Geometry check sheet. Reference: the model listing, model coordinates, mm. Face numbers are marked on the shaded views. Give positions to 0.01 mm unless a question says otherwise; leave off trailing zeros. Loops run counter-clockwise (first coordinate to the right, second up) from the corner with the lowest first, then second, coordinate; pieces in that order, holes last. Notation, with made-up numbers: (-36.5, -19.75) -> (-32.5, -19.75) arc R25 cw to (-32.5, -1.75) -> close; hole circle Ø1 at (-7, 58.25). An arc over 180 degrees is marked (long way). Answer as a JSON object with one key per item and string values.
from build123d import *

# Parameters (mm, degrees)
F0_W      = 59.395711869
F0_H      = 250.2426505089
F1_DEPTH  = 67.4364492297
F2_R      = 17.4264129212
F3_DEPTH  = 222.8358983994
F4_W      = 62.507584691
F4_H      = 75.5731239915
F5_DEPTH  = 227.648139
F6_W      = 115.2810156345
F6_H      = 19.8185071349
F7_DEPTH  = 53.9569482207
F8_W      = 67.4364492297
F8_H      = 12.6657411456
F8_H_2    = 15.0272101164
F9_DEPTH  = 599.2090702057
F10_R     = 17.5883740648
F11_DEPTH = 151.8874019384
F12_R     = 10.9031193455
F13_DEPTH = 69.4709941745


# Not quite as in the source:
# - a feature names something its author has since deleted; it is built from what else it names


with BuildPart() as f1:
    # F0 (on Front) → F1 (new body)
    with BuildSketch(Plane.XZ):
        Rectangle(F0_W, F0_H)
    extrude(amount=F1_DEPTH)

    # F2 (on face) → F3 (join)
    with BuildSketch(Plane.XY.offset(125.1213252544)):
        with Locations((0, -33.2162864506)):
            Circle(F2_R)
    extrude(amount=-F3_DEPTH)

    # F4 (on face) → F5 (join)
    with BuildSketch(Plane(origin=(-29.6978559345, 0, 0), x_dir=(0, -1, 0), z_dir=(-1, 0, 0))):
        with Locations((36.1826568842, 0)):
            Rectangle(F4_W, F4_H)
    extrude(amount=F5_DEPTH)

    # F6 (on face) → F7 (join)
    with BuildSketch(Plane(origin=(0, -4.9288645387, 0), x_dir=(-1, 0, 0), z_dir=(0, 1, 0))):
        with Locations((168.05139184, 0)):
            Rectangle(F6_W, F6_H)
    extrude(amount=F7_DEPTH)

    # F8 (on face) → F9 (join)
    with BuildSketch(Plane.YZ.offset(29.6978559345)):
        with Locations((-33.7182246149, -118.7884546816)):
            Rectangle(F8_W, F8_H)
        with Locations((-33.7182246149, 117.6077201962)):
            Rectangle(F8_W, F8_H_2)
    extrude(amount=F9_DEPTH)

    # F10 (on face) → F11 (join)
    with BuildSketch(Plane(origin=(-257.3459949344, 0, 0), x_dir=(0, -1, 0), z_dir=(-1, 0, 0))):
        with Locations((40.5630767345, 0)):
            Circle(F10_R)
    extrude(amount=F11_DEPTH)

    # F12 (on face) → F13 (join)
    with BuildSketch(Plane(origin=(0, 0, -9.9092535675), x_dir=(1, 0, 0), z_dir=(0, 0, -1))):
        with Locations((-176.2370765209, -20.2873200178)):
            Circle(F12_R)
    extrude(amount=F13_DEPTH)


solid = f1.part
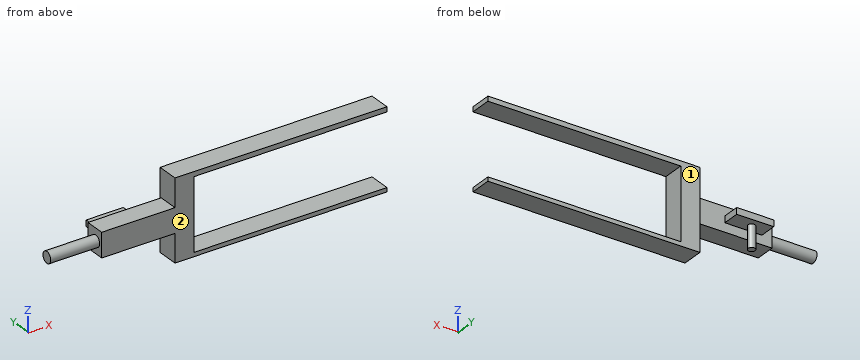
1) Section check B-B on x = -147.5. Record the cut outline in (y, z), plus the area to 3 significant figures.
Geometry check:
{"outline": "(-67.44, -37.79) -> (-4.93, -37.79) -> (-4.93, -9.91) -> (49.03, -9.91) -> (49.03, 9.91) -> (-4.93, 9.91) -> (-4.93, 37.79) -> (-67.44, 37.79) -> close", "area": "5,790 mm2"}
2) Section check C-C on z = 0. Record the cut outline in (x, y), plus the area to 3 significant figures.
Geometry check:
{"outline": "(-409.23, -58.15) -> (-257.35, -58.15) -> (-257.35, -67.44) -> (29.7, -67.44) -> (29.7, 0) -> (-29.7, 0) -> (-29.7, -4.93) -> (-110.41, -4.93) -> (-110.41, 49.03) -> (-225.69, 49.03) -> (-225.69, -4.93) -> (-257.35, -4.93) -> (-257.35, -22.97) -> (-409.23, -22.97) -> close", "area": "29,800 mm2"}
3) Depth check by flat-ended pin: P1, Ø8, axis at x = -149, y = -18.5, coming from the -Z side; P2, Ø4, axis at y = -30, z = 67.5, coming from the -X side; P3, Ø22, axis at y = 22, z = 3, coming from the +X side. Enter the tip coordinate at first touch or a pass-through.
Geometry check:
{"P1": "stops at z = -37.79", "P2": "stops at x = -29.7", "P3": "stops at x = -110.41"}
4) Section check D-D on z = -52. Record the cut outline in (x, y), plus the area to 3 significant figures.
Geometry check:
{"outline": "circle Ø21.81 at (-176.24, 20.29); (-29.7, -67.44) -> (29.7, -67.44) -> (29.7, 0) -> (-29.7, 0) -> close", "area": "4,380 mm2"}
5) Section check A-A on x = 234. Record the cut outline in (y, z).
Geometry check:
{"outline": "(-67.44, -125.12) -> (0, -125.12) -> (0, -112.46) -> (-67.44, -112.46) -> close; (-67.44, 110.09) -> (0, 110.09) -> (0, 125.12) -> (-67.44, 125.12) -> close"}
6) Draft check along Y on the marked faces 1 and 2. Enter one of: pulls with the +Y half, pulls with the -Y half, needs draft (parallel to the pull), parting line crosses it, or undercut.
Geometry check:
{"face 1": "pulls with the +Y half", "face 2": "pulls with the -Y half"}
7) Material ranges on line 1 along Z through (x, y) = (167, -44); line 2 along Z through (x, y) = (-160.5, -53.5); line 3 along Y through (x, z) = (-36.5, -32.5), recorded low to high. Write a range as from..to.
Geometry check:
{"line 1": "z = -125.12..-112.46, 110.09..125.12", "line 2": "z = -37.79..37.79", "line 3": "y = -67.44..-4.93"}
